Can you work these out from the model? Positions are in its coordinate system, mm. Face numbers are marked on the shaded views. A direction names the side the tool comes from. Coordinates: 2 decimals unless noted, no trailing zeros. Loops run counter-clockwise (first coordinate to the right, second up) from the corner with the lowest first, then second, coordinate; pieces in that order, holes last. Notation, with made-up numbers: (47.25, 49.25) -> (64.25, 49.25) arc R25 ccw to (64.25, 81.25) -> close; hole circle Ø11 at (87, 5.5). An arc over 180 degrees is marked (long way). Put each result on its own line as item: value. Start each with the question number.
Item 1: If we section it at B-B on x = 0: Please give me the cut outline in (y, z), plus the area to 3 significant figures.
Item 2: If we section it at D-D on z = 16: Please give me the cut outline in (x, y).
Item 3: For the marked faces 3 and 4, which set-ups out of +Z, -Z, +X, -X, +Y, -Y let a thin tool reach every point of the face, with its end or its side?
Item 4: Will these pins go through, and if not, where does the flat tip stop? P1, Ø6, axis at x = 18, z = -23, coming from the -Y side; P2, Ø3, axis at y = 135, z = 16, coming from the -X side; P3, Ø1.3, axis at y = 255.5, z = 6, coming from the +X side.
Item 5: If we section it at A-A on z = 0: Please give me the cut outline in (x, y).
Item 6: We'd pull the mould along X, two halves only. Please class the marked faces 1 and 2: pulls with the +X half, pulls with the -X half, needs draft (parallel to the pull), parting line crosses it, or undercut.
Item 7: Please list where these lines run through material, in increasing order: L1, parallel to Y at x = 16, z = 20.5; L2, parallel to Y at x = -33, z = -3.5; L3, parallel to X at y = 201, z = -1. Write a range as from..to.
Item 8: If we section it at C-C on y = 69: Please give me the cut outline in (x, z), plus the area to 3 significant figures.
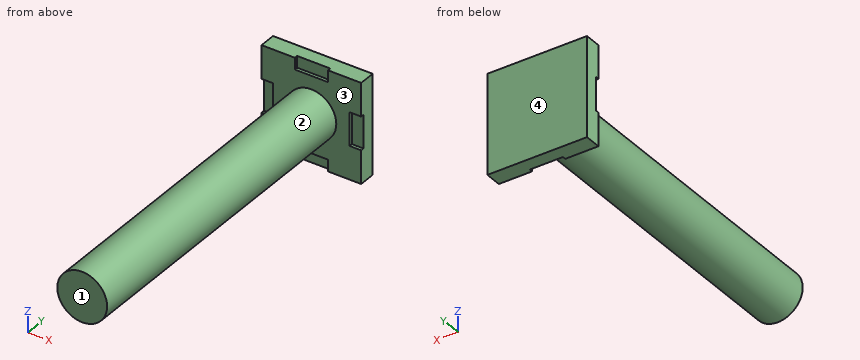
```python
from build123d import *

# Parameters (mm, degrees)
SKETCH1_R           = 19.05
BOSS_EXTRUDE1_DEPTH = 254
SKETCH5_W           = 76.2
SKETCH5_H           = 76.2
BOSS_EXTRUDE3_DEPTH = 12.7
SKETCH6_W           = 8.89
SKETCH6_H           = 25.4
SKETCH6_W_2         = 25.4
SKETCH6_H_2         = 8.89
CUT_EXTRUDE1_DEPTH  = 2.54


with BuildPart() as part:
    # Sketch1 → Boss-Extrude1 (new body)
    with BuildSketch(Plane(origin=(0, 0, 0), x_dir=(1, 0, 0), z_dir=(0, 1, 0))):
        Circle(SKETCH1_R)
    extrude(amount=BOSS_EXTRUDE1_DEPTH)

    # Sketch5 → Boss-Extrude3 (add)
    with BuildSketch(Plane(origin=(0, 254, 0), x_dir=(1, 0, 0), z_dir=(0, 1, 0))):
        Rectangle(SKETCH5_W, SKETCH5_H)
    extrude(amount=BOSS_EXTRUDE3_DEPTH)

    # Sketch6 → Cut-Extrude1 (cut)
    with BuildSketch(Plane.XZ.offset(-254)):
        with Locations((-33.655, 0)):
            Rectangle(SKETCH6_W, SKETCH6_H)
        with Locations((0, 33.655)):
            Rectangle(SKETCH6_W_2, SKETCH6_H_2)
        with Locations((33.655, 0)):
            Rectangle(SKETCH6_W, SKETCH6_H)
        with Locations((0, -33.655)):
            Rectangle(SKETCH6_W_2, SKETCH6_H_2)
    extrude(amount=-CUT_EXTRUDE1_DEPTH, mode=Mode.SUBTRACT)


solid = part.part
```
Solutions:
1. outline: (0, -19.05) -> (254, -19.05) -> (254, -29.21) -> (256.54, -29.21) -> (256.54, -38.1) -> (266.7, -38.1) -> (266.7, 38.1) -> (256.54, 38.1) -> (256.54, 29.21) -> (254, 29.21) -> (254, 19.05) -> (0, 19.05) -> close
1. area: 10,600 mm^2
2. outline: (-38.1, 254) -> (-10.34, 254) -> (-10.34, 0) -> (10.34, 0) -> (10.34, 254) -> (38.1, 254) -> (38.1, 266.7) -> (-38.1, 266.7) -> close
3. face 3: -Y
3. face 4: +Z, -Z, +X, -X, +Y
4. P1: y = 254
4. P2: x = -12.36
4. P3: x = 29.21
5. outline: (-38.1, 256.54) -> (-29.21, 256.54) -> (-29.21, 254) -> (-19.05, 254) -> (-19.05, 0) -> (19.05, 0) -> (19.05, 254) -> (29.21, 254) -> (29.21, 256.54) -> (38.1, 256.54) -> (38.1, 266.7) -> (-38.1, 266.7) -> close
6. face 1: needs draft
6. face 2: parting line crosses it
7. L1: 254..266.7
7. L2: 256.54..266.7
7. L3: -19.02..19.02
8. outline: circle Ø38.1 at (0, 0)
8. area: 1,140 mm^2
